from build123d import *

# Parameters (mm, degrees)
SKETCH_2_W         = 62
SKETCH_2_H         = 10
SKETCH_2_R         = 0.5
EXTRUDE_1_DEPTH    = 4
HOLE_WIZARD_M5_1_D = 4.2
HOLE_WIZARD_M5_2_D = 4.2
CHAMFER_1_SIZE     = 0.5


with BuildPart() as part:
    # 草图2 → 凸台-拉伸1 (new, symmetric)
    with BuildSketch(Plane.XY):
        Rectangle(SKETCH_2_W, SKETCH_2_H)
        with Locations((-26, 0)):
            Circle(SKETCH_2_R, mode=Mode.SUBTRACT)
        with Locations((26, 0)):
            Circle(SKETCH_2_R, mode=Mode.SUBTRACT)
    extrude(amount=EXTRUDE_1_DEPTH, both=True)

    # M5 螺纹孔1 (through all)
    with Locations(Plane.XY.offset(4)):
        with Locations((0, 0), (-26, 0), (26, 0)):
            Hole(HOLE_WIZARD_M5_1_D / 2)

    # M5 螺纹孔2 (through all)
    with Locations(Plane(origin=(0, 5, 0), x_dir=(1, 0, 0), z_dir=(0, 1, 0))):
        with Locations((16, 0), (-16, 0)):
            Hole(HOLE_WIZARD_M5_2_D / 2)

    # 倒角1
    chamfer_1_edges = [part.edges().sort_by_distance(p)[0] for p in [
        (0, -5, 4),
        (31, 0, 4),
        (0, 5, 4),
        (31, 0, -4),
        (0, -5, -4),
        (-31, 0, -4),
        (0, 5, -4),
        (-31, 0, 4),
        (31, 5, 0),
        (31, -5, 0),
        (-31, -5, 0),
        (-31, 5, 0),
    ]]
    chamfer(chamfer_1_edges, length=CHAMFER_1_SIZE)


solid = part.part
Source: CAD feature listing. Evaluate the final solid. Frame: model axes, mm. Coordinates: 2 decimals unless noted, no trailing zeros. Write each loop counter-clockwise with the first axis right and the second up, starting at its lowest first coordinate (ties: lowest second). Pieces come first, ordered by that corner, then holes. Notation, with made-up numbers: M -10,49 L 12,49 A37 ccw 12,87 Z; hole C 67,30.5 d6. An arc over 180 degrees is marked long. Use a Markdown table: item, result.
1) Section B-B, the plane x = 0. Output: boundary loops of the cut face in (y, z).
Conclusion:
| item | result |
|---|---|
| outline | M -5,-3.5 L -4.5,-4 L -2.1,-4 L -2.1,4 L -4.5,4 L -5,3.5 Z; M 2.1,-4 L 4.5,-4 L 5,-3.5 L 5,3.5 L 4.5,4 L 2.1,4 Z |
2) Section C-C, the plane z = 2.75. Output: boundary loops of the cut face in (x, y).
Conclusion:
| item | result |
|---|---|
| outline | M -31,-4.5 L -30.5,-5 L 30.5,-5 L 31,-4.5 L 31,4.5 L 30.5,5 L -30.5,5 L -31,4.5 Z; hole C -26,0 d4.2; hole C 0,0 d4.2; hole C 26,0 d4.2 |
3) Ray query, L1, parallel to Y at x = 26, z = -0.25; L2, parallel to X at y = -1.75, z = -1.5; L3, parallel to X at y = -3.75, z = -0.25. Return the intervals inside material, ascending.
Conclusion:
| item | result |
|---|---|
| L1 | y = -5 to -2.1, 2.1 to 5 |
| L2 | x = -31 to -27.16, -24.84 to -17.47, -14.53 to -1.16, 1.16 to 14.53, 17.47 to 24.84, 27.16 to 31 |
| L3 | x = -31 to -18.09, -13.91 to 13.91, 18.09 to 31 |
4) Mould query, pull axis Z, two halves, no side actions, for faces 1 (the cylindrical face through (28.1, 0.09, -0.06)), 2 (the cylindrical face through (18.1, -0.07, -0.09)), 3 (the cylindrical face through (-13.9, -0.07, -0.09)), 4 (the flat face through (0, 3, -4)). Classes: pulls with the +Z half, pulls with the -Z half, needs draft (parallel to the pull), parting line crosses it, or undercut.
Conclusion:
| item | result |
|---|---|
| face 1 | needs draft |
| face 2 | undercut |
| face 3 | undercut |
| face 4 | pulls with the -Z half |
5) Section A-A, the plane z = 0. Output: boundary loops of the cut face in (x, y), then the cut area to 3 significant figures.
Conclusion:
| item | result |
|---|---|
| outline | M -31,-4.5 L -30.5,-5 L -18.1,-5 L -18.1,5 L -30.5,5 L -31,4.5 Z; M -13.9,-5 L 13.9,-5 L 13.9,5 L -13.9,5 Z; M 18.1,-5 L 30.5,-5 L 31,-4.5 L 31,4.5 L 30.5,5 L 18.1,5 Z; hole C -26,0 d4.2; hole C 0,0 d4.2; hole C 26,0 d4.2 |
| area | 494 mm^2 |
6) Section D-D, the plane x = 16. Output: boundary loops of the cut face in (y, z), then the cut area to 3 significant figures.
Conclusion:
| item | result |
|---|---|
| outline | M -5,-3.5 L -4.5,-4 L 4.5,-4 L 5,-3.5 L 5,-2.1 L -5,-2.1 Z; M -5,2.1 L 5,2.1 L 5,3.5 L 4.5,4 L -4.5,4 L -5,3.5 Z |
| area | 37.5 mm^2 |
7) First-contact query: pin 1 Ø5 at (x, y) = (-26, 0) entering from +Z. Flat tip, straight axial feed; report the tip coordinate or a pass-through.
Conclusion:
| item | result |
|---|---|
| pin 1 | stops at z = 4 |
